Input: part model. Units: mm. Frame: model coordinates. Face numbers are marked on the shaded views. Round coordinates to 2 decimals unless told otherwise and drop trailing zeros. Loops run counter-clockwise (first coordinate to the right, second up) from the corner with the lowest first, then second, coordinate; pieces in that order, holes last. Notation, with made-up numbers: (18, 83.25) -> (52, 83.25) arc R15 ccw to (52, 96.25) -> close; hole circle Ø5 at (-21.75, 14.25). An arc over 180 degrees is marked (long way). Answer as a JSON object with one key per item and string values. Group by question number.
Item 1: Section query C-C on z = -37. Return loops of the section in (x, y), and give its area (3 significant figures).
Item 2: Pin query (flat end, axial travel): pin 1 (5 mm diameter, centred on x = 18, z = -23, fed in from -Y); pin 2 (3 mm diameter, centred on x = 15.5, z = -40, fed in from +Y); pin 3 (2.5 mm diameter, centred on x = 12.5, z = -4, fed in from +Y). Return the tip coordinate at first contact, or that it passes through.
Item 3: Draft query along X for the marked faces 1, 2 and 3. Return one class per face: released by +X, released by -X, zero draft, split by the parting line, or undercut.
Item 4: Section query B-B on x = 12.5. Return loops of the section in (y, z).
Item 5: Material intervals for line 1 (Z direction, x = 12.5, y = 1.2); line 2 (X direction, y = 1.3, z = -4); line 3 (X direction, y = 2.2, z = -42), sorted ascending. Write a range as [from, to].
Item 6: Section query D-D on x = 22.25. Return loops of the section in (y, z).
Item 7: Section query A-A on z = -4. Return loops of the section in (x, y), and give its area (3 significant figures).
Autodesk Inventor part; units mm, degrees
ref_plane "YZ Plane" through (0, 0, 0) normal (1, 0, 0) x (0, 1, 0)
ref_plane "XZ Plane" through (0, 0, 0) normal (0, 1, 0) x (-1, 0, 0)
ref_plane "XY Plane" through (0, 0, 0) normal (0, 0, 1) x (1, 0, 0)
sketch "Sketch1" plane through (0, 0, 0) normal (0, 1, 0) x (-1, 0, 0)
  line L0 (0, 0) -> (-25, 0)
  line L1 (-25, 0) -> (-25, -46.5)
  line L2 (-25, -46.5) -> (0, -46.5)
  line L3 (0, -46.5) -> (0, 0)
  dimension "d0" = 25
  dimension "d1" = 46.5
extrude "Extrusion1" add sketch "Sketch1" along normal blind 2
sketch "Sketch2" plane through (0, 2, 0) normal (0, 1, 0) x (1, 0, 0)
  line L0 (25, 46.5) -> (0, 46.5)
  line L1 (0, 46.5) -> (6, 46.5)
  line L2 (6, 46.5) -> (6, 36.5)
  line L3 (6, 36.5) -> (0, 36.5)
  line L4 (0, 36.5) -> (0, 46.5)
  line L5 (25, 46.5) -> (19, 46.5)
  line L6 (19, 46.5) -> (19, 36.5)
  line L7 (19, 36.5) -> (25, 36.5)
  line L8 (25, 36.5) -> (25, 46.5)
  point P0 (0, 0)
  dimension "d4" = 6
  dimension "d5" = 10
  dimension "d6" = 6
extrude "Extrusion2" add sketch "Sketch2" along normal blind 2
sketch "Sketch3" plane through (0, 2, 0) normal (0, 1, 0) x (1, 0, 0)
  line L0 (0, 0) -> (25, 0)
  line L1 (25, 0) -> (25, 36.5)
  point P0 (12.5, 4)
  dimension "d9" = 4
  dimension "d10" = 12.5
hole "Hole1" at (12.5, 2, -4) direction (0, -1, 0) diameter 3.2 end through all
properties part number "mlx_mount_2mm"
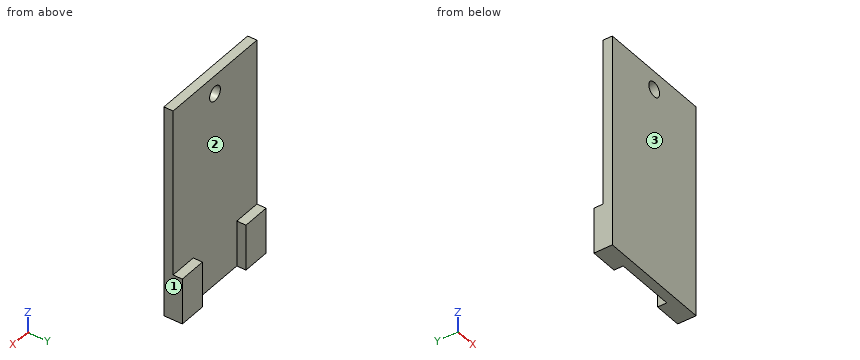
Solved:
{
 "1": {"outline": "(0, 0) -> (25, 0) -> (25, 4) -> (19, 4) -> (19, 2) -> (6, 2) -> (6, 4) -> (0, 4) -> close", "area": "74.0 mm²"},
 "2": {"pin 1": "y = 0", "pin 2": "y = 2", "pin 3": "through"},
 "3": {"face 1": "released by +X", "face 2": "undercut", "face 3": "zero draft"},
 "4": {"outline": "(0, -46.5) -> (2, -46.5) -> (2, -5.6) -> (0, -5.6) -> close; (0, -2.4) -> (2, -2.4) -> (2, 0) -> (0, 0) -> close"},
 "5": {"line 1": "[-46.5, -5.6], [-2.4, 0]", "line 2": "[0, 10.9], [14.1, 25]", "line 3": "[0, 6], [19, 25]"},
 "6": {"outline": "(0, -46.5) -> (4, -46.5) -> (4, -36.5) -> (2, -36.5) -> (2, 0) -> (0, 0) -> close"},
 "7": {"outline": "(0, 0) -> (10.9, 0) -> (10.9, 2) -> (0, 2) -> close; (14.1, 0) -> (25, 0) -> (25, 2) -> (14.1, 2) -> close", "area": "43.6 mm²"}
}
